Input: part model. Units: mm. Frame: model coordinates. Face numbers are marked on the shaded views. Coordinates: 2 decimals unless noted, no trailing zeros. Loops run counter-clockwise (first coordinate to the right, second up) from the corner with the lowest first, then second, coordinate; pieces in that order, holes last.
Item 1: Contact query for flat-ended pins moving along their axis: P1, Ø12, axis at x = -68, z = -61.5, coming from the -Y side; P2, Ø2, axis at y = 11, z = -21.5, coming from the +X side; P3, Ø8, axis at x = 65, z = -37, coming from the +Y side; P4, Ø13.5, axis at x = -4.5, z = -89.5, coming from the +Y side. Output: stop coordinate, or through.
Item 2: Ray query, line 1 along X through (y, z) = (-85.85, -85.67); line 2 along X through (y, z) = (11.5, -60); line 3 along X through (y, z) = (83.2, -8.25). Return the intervals inside material, ascending.
Item 3: Section A-A on x = 68. Return loops of the section in (y, z), and give its area (3 significant figures).
Item 4: Section C-C on z = -73. Return loops of the section in (x, y).
Item 5: Section B-B on y = -67. Return loops of the section in (x, z).
Item 6: Pull-direction query (Y, two-part tool) for the marked faces 1, 2 and 3; classes: released by +Y, released by -Y, zero draft, split by the parting line, or undercut.
```python
from build123d import *

# Parameters (mm, degrees)
SKETCH1_R                 = 93.40293561
SKETCH1_R_2               = 83.40293561
BOSS_EXTRUDE1_DEPTH       = 93.92
BOSS_EXTRUDE3_DEPTH       = 93.92
CUT_EXTRUDE1_REACH        = 231.001
SKETCH2_W                 = 34
SKETCH2_H                 = 69
CUT_EXTRUDE2_START        = -6.472936
SKETCH3_W                 = 34
SKETCH3_H                 = 12.46
CUT_EXTRUDE2_DEPTH        = 6.472936
M5_CLEARANCE_HOLE1_D      = 5.8
M5_CLEARANCE_HOLE1_DEPTH  = 170.33393561
M5_CLEARANCE_HOLE1_TIP    = 1.742495795
SKETCH8_W                 = 4.19
SKETCH8_H                 = 3.07
CUT_EXTRUDE3_DEPTH        = 12.46
M6_CLEARANCE_HOLE1_REACH  = 219.335
M6_CLEARANCE_HOLE1_BORE_R = 1.5


with BuildPart() as part:
    # Sketch1 → Boss-Extrude1 (new body)
    with BuildSketch(Plane.XY):
        Circle(SKETCH1_R)
        Circle(SKETCH1_R_2, mode=Mode.SUBTRACT)
    extrude(amount=-BOSS_EXTRUDE1_DEPTH)

    # Sketch7 → Boss-Extrude3 (add)
    with BuildSketch(Plane.XY):
        with BuildLine():
            Line((-17, -81.652003456), (17, -81.652003456))
            ThreePointArc((17, -81.652003456), (0, -83.40293561), (-17, -81.652003456))
        make_face()
    extrude(amount=-BOSS_EXTRUDE3_DEPTH)

    # Sketch2 → Cut-Extrude1 (cut, up to next)
    with BuildSketch(Plane(origin=(0, -93.40293561, 0), x_dir=(-1, 0, 0), z_dir=(0, -1, 0)), mode=Mode.PRIVATE) as cut_extrude1_sk1:
        with Locations((0, 46.96)):
            Rectangle(SKETCH2_W, SKETCH2_H)
    cut_extrude1_tool1 = extrude(cut_extrude1_sk1.sketch, amount=-CUT_EXTRUDE1_REACH, mode=Mode.PRIVATE) & part.part
    add(cut_extrude1_tool1.solids().sort_by_distance((0, -93.402936, -46.96))[0], mode=Mode.SUBTRACT)

    # Sketch3 → Cut-Extrude2 (cut)
    with BuildSketch(Plane(origin=(0, -93.40293561, 0), x_dir=(-1, 0, 0), z_dir=(0, -1, 0)).offset(CUT_EXTRUDE2_START)):
        with Locations((0, 87.69)):
            Rectangle(SKETCH3_W, SKETCH3_H)
        with Locations((0, 6.23)):
            Rectangle(SKETCH3_W, SKETCH3_H)
    extrude(amount=CUT_EXTRUDE2_DEPTH, mode=Mode.SUBTRACT)

    # M5 Clearance Hole1
    with Locations(Plane(origin=(-7.5, -86.93, -8.25), x_dir=(0, 0, -1), z_dir=(0, -1, 0))):
        with Locations((0, 0), (0, 15), (77.42, 0), (77.42, 15)):
            Hole(M5_CLEARANCE_HOLE1_D / 2, depth=M5_CLEARANCE_HOLE1_DEPTH)
            with Locations((0, 0, -(M5_CLEARANCE_HOLE1_DEPTH + M5_CLEARANCE_HOLE1_TIP / 2))):  # 118° drill point
                Cone(0, M5_CLEARANCE_HOLE1_D / 2, M5_CLEARANCE_HOLE1_TIP, mode=Mode.SUBTRACT)

    # Sketch8 → Cut-Extrude3 (cut)
    with BuildSketch(Plane.XY):
        with Locations((0, -85.395)):
            Rectangle(SKETCH8_W, SKETCH8_H)
    extrude(amount=-CUT_EXTRUDE3_DEPTH, mode=Mode.SUBTRACT)

    # M6 Clearance Hole1 bore (on position points) → M6 Clearance Hole1 (cut, up to next)
    with BuildSketch(Plane(origin=(93.40293561, 0, -60.116902822), x_dir=(0, 0, 1), z_dir=(1, 0, 0)), mode=Mode.PRIVATE) as m6_clearance_hole1_sk1:
        Circle(M6_CLEARANCE_HOLE1_BORE_R)
    m6_clearance_hole1_tool1 = extrude(m6_clearance_hole1_sk1.sketch, amount=-M6_CLEARANCE_HOLE1_REACH, mode=Mode.PRIVATE) & part.part
    # M6 Clearance Hole1 bore (on position points) → M6 Clearance Hole1 (cut, up to next)
    with BuildSketch(Plane(origin=(93.40293561, 0, -60.116902822), x_dir=(0, 0, 1), z_dir=(1, 0, 0)), mode=Mode.PRIVATE) as m6_clearance_hole1_sk2:
        with Locations((10, 0)):
            Circle(M6_CLEARANCE_HOLE1_BORE_R)
    m6_clearance_hole1_tool2 = extrude(m6_clearance_hole1_sk2.sketch, amount=-M6_CLEARANCE_HOLE1_REACH, mode=Mode.PRIVATE) & part.part
    add(m6_clearance_hole1_tool1.solids().sort_by_distance((93.402936, 0, -60.116903))[0], mode=Mode.SUBTRACT)
    add(m6_clearance_hole1_tool2.solids().sort_by_distance((93.402936, 0, -50.116903))[0], mode=Mode.SUBTRACT)


solid = part.part
```
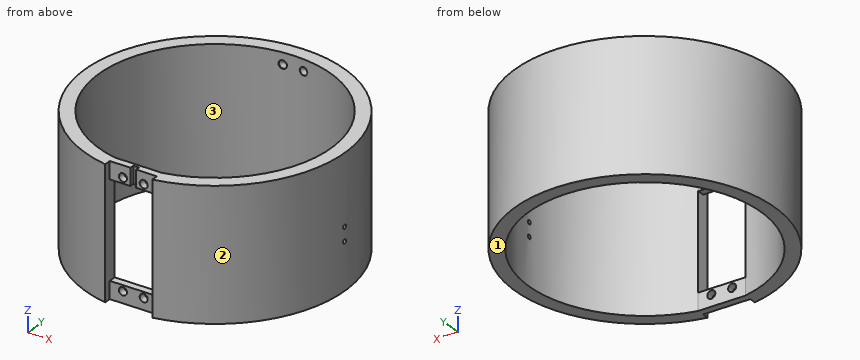
Results found:
1. P1: stops at y = -69.86
1. P2: stops at x = 92.87
1. P3: stops at y = 70.73
1. P4: stops at y = 93.4
2. line 1: x = -36.8 to -10.4, -4.6 to 4.6, 10.4 to 36.8
2. line 2: x = -92.69 to -82.61, 82.61 to 92.69
2. line 3: x = -42.45 to -10.4, 10.4 to 42.45
3. outline: (-64.03, -93.92) - (-48.29, -93.92) - (-48.29, 0) - (-64.03, 0) - close; (48.29, -93.92) - (64.03, -93.92) - (64.03, 0) - (48.29, 0) - close
3. area: 2,960 mm2
4. outline: (-17, -91.84) - (-17, -81.65) arc R83.4 cw (long way) to (17, -81.65) - (17, -91.84) arc R93.4 ccw (long way) to start
5. outline: (-65.08, -93.92) - (-49.67, -93.92) - (-49.67, 0) - (-65.08, 0) - close; (49.67, -93.92) - (65.08, -93.92) - (65.08, 0) - (49.67, 0) - close
6. face 1: zero draft
6. face 2: split by the parting line
6. face 3: undercut
